Autodesk Inventor part; units mm, degrees
ref_plane "YZ Plane" through (0, 0, 0) normal (1, 0, 0) x (0, 1, 0)
ref_plane "XZ Plane" through (0, 0, 0) normal (0, 1, 0) x (-1, 0, 0)
ref_plane "XY Plane" through (0, 0, 0) normal (0, 0, 1) x (1, 0, 0)
sketch "Sketch1" plane through (0, 0, 0) normal (0, 1, 0) x (-1, 0, 0)
  circle A0 centre (0, 0) radius 39.5
  circle A1 centre (0, 0) radius 10
  circle A2 centre (0, 0) radius 29
  circle A3 centre (29, 0) radius 2.75
  circle A4 centre (0, 29) radius 2.75
  circle A5 centre (-29, 0) radius 2.75
  circle A6 centre (0, -29) radius 2.75
  dimension "d2" = 58
  dimension "d0" = 79
  dimension "d1" = 20
  dimension "d3" = 5.5
  dimension "d6" = 360
extrude "Extrusion1" add sketch "Sketch1" along normal blind 10 contours A0 | A1 | A3 A2 A6 A5 A4
sketch "Sketch3" plane through (0, 10, 0) normal (0, 1, 0) x (1, 0, 0)
  line L0 (-34.5, 50.157) -> (-34.5, -49.8555)
  circle A0 centre (0, 0) radius 39.5
  point P0 (-34.5, -19.2354)
  point P1 (-34.5, 19.2354)
  dimension "d18" = 5
extrude "Extrusion3" cut sketch "Sketch3" along normal through all both and the other way through all contours L0 A0 picked at (-35.5583, 3.956)
sketch "Sketch4" plane through (0, 0, 0) normal (0, -1, 0) x (1, 0, 0)
  circle A0 centre (0, 0) radius 9.2075
  dimension "d21" = 18.415
extrude "Extrusion4" cut sketch "Sketch4" against normal through all
sketch "Sketch5" plane through (0, 0, 0) normal (0, -1, 0) x (1, 0, 0)
  line L0 (33, -2.3094) -> (29, -4.6188)
  line L1 (29, -4.6188) -> (25, -2.3094)
  line L2 (25, -2.3094) -> (25, 2.3094)
  line L3 (25, 2.3094) -> (29, 4.6188)
  line L4 (29, 4.6188) -> (33, 2.3094)
  line L5 (33, 2.3094) -> (33, -2.3094)
  circle A0 centre (29, 0) radius 2.75
  line L6 (-2.3094, 33) -> (2.3094, 33)
  line L7 (4.6188, 29) -> (2.3094, 25)
  line L8 (2.3094, 25) -> (-2.3094, 25)
  line L9 (-2.3094, 25) -> (-4.6188, 29)
  circle A1 centre (0, 29) radius 2.75
  line L10 (2.3094, 33) -> (4.6188, 29)
  line L11 (-4.6188, 29) -> (-2.3094, 33)
  line L12 (-33, -2.3094) -> (-33, 2.3094)
  line L13 (-29, 4.6188) -> (-25, 2.3094)
  line L14 (-25, 2.3094) -> (-25, -2.3094)
  line L15 (-25, -2.3094) -> (-29, -4.6188)
  circle A2 centre (-29, 0) radius 2.75
  line L16 (-33, 2.3094) -> (-29, 4.6188)
  line L17 (-29, -4.6188) -> (-33, -2.3094)
  line L18 (2.3094, -33) -> (-2.3094, -33)
  line L19 (-4.6188, -29) -> (-2.3094, -25)
  line L20 (-2.3094, -25) -> (2.3094, -25)
  line L21 (2.3094, -25) -> (4.6188, -29)
  circle A3 centre (0, -29) radius 2.75
  line L22 (-2.3094, -33) -> (-4.6188, -29)
  line L23 (4.6188, -29) -> (2.3094, -33)
  point P0 (0, 0)
  point P1 (0, 0)
  point P2 (33, 0)
  point P3 (0, 33)
  point P4 (-33, 0)
  point P5 (0, -33)
  dimension "d27" = 360
extrude "Extrusion5" cut sketch "Sketch5" against normal blind 5
properties part number "Adapter Plate"
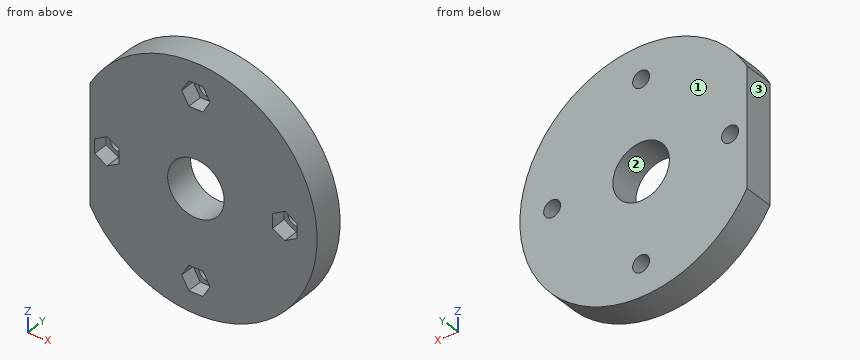
Geometry check sheet. Reference: the model listing, model coordinates, mm. Face numbers are marked on the shaded views. Coordinates: 2 decimals unless noted, no trailing zeros. Order: outer loops, then holes, each group sorted by start corner. A loop starts at its lowest first (then second) coordinate and runs counter-clockwise, first axis right, second up. Notation, with made-up numbers: M 50,-35.5 L 63,-35.5 A20 cw 63,-13.5 Z; hole C 19,58 d8. An arc over 180 degrees is marked long. Use CSV: the item, a comma, the result in double quotes.
Item 1: Cross-section at B-B on x = 28. Record the cut outline in (y, z).
Returned:
outline,"M 0,-27.86 L 10,-27.86 L 10,-2.56 L 5,-2.56 L 5,-4.04 L 0,-4.04 Z; M 0,4.04 L 5,4.04 L 5,2.56 L 10,2.56 L 10,27.86 L 0,27.86 Z"
Item 2: Mould release check, pull along X, two halves, no side actions. Record for the marked faces 1, 2 and 3: pulls with the +X half, pulls with the -X half, needs draft (parallel to the pull), parting line crosses it, or undercut.
Returned:
face 1,"needs draft"
face 2,"undercut"
face 3,"pulls with the -X half"
Item 3: Cross-section at A-A on y = 6. Give the number of separate pieces and of enclosed holes in the cut face, then the cut area to 3 significant figures.
Returned:
separate pieces,"1"
enclosed holes,"5"
area,"4,410 mm2"
Item 4: Gauge pin test, flat ends, axial feed: pin 1 Ø6.5 at (x, z) = (-1, -27.5) entering from -Y; pin 2 Ø1 at (y, z) = (8, 28.5) entering from -X; pin 3 Ø2 at (x, y) = (24, 7.5) entering from +Z; pin 4 Ø3 at (x, y) = (-9, 1) entering from +Z. Record the tip position at first contact, or that the pin passes through.
Returned:
pin 1,"stops at y = 0"
pin 2,"stops at x = -27.86"
pin 3,"stops at z = 32.11"
pin 4,"stops at z = 38.78"
Item 5: Cross-section at C-C on x = 16. Record the cut outline in (y, z), then the cut area to 3 significant figures.
Returned:
outline,"M 0,-36.11 L 10,-36.11 L 10,36.11 L 0,36.11 Z"
area,"722 mm2"
Item 6: Thickness scan on line 1 along Z through (x, y) = (0, 7.4); line 2 along Z through (x, y) = (4, 1.75); line 3 along Z through (x, y) = (-6, 7.75). Record the ranges inside material, lowest first.
Returned:
line 1,"z = -39.5 to -31.75, -26.25 to -9.21, 9.21 to 26.25, 31.75 to 39.5"
line 2,"z = -39.3 to -30.07, -27.93 to -8.29, 8.29 to 27.93, 30.07 to 39.3"
line 3,"z = -39.04 to -6.98, 6.98 to 39.04"
Item 7: Cross-section at D-D on z = 17. Record the cut outline in (x, y), then the cut area to 3 significant figures.
Returned:
outline,"M -34.5,0 L 35.65,0 L 35.65,10 L -34.5,10 Z"
area,"702 mm2"
